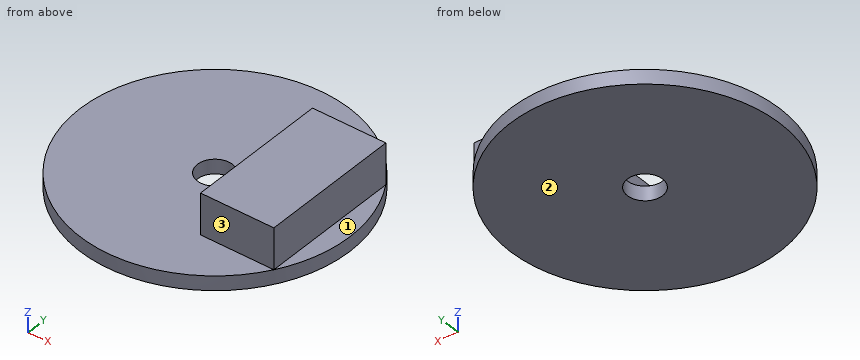
from build123d import *

# Parameters (mm, degrees)
SKETCH1_R           = 11.5
BOSS_EXTRUDE1_DEPTH = 1.23
SKETCH2_W           = 6.25
SKETCH2_H           = 12.059402844
BOSS_EXTRUDE2_DEPTH = 3.5
SKETCH3_R           = 1.5
CUT_EXTRUDE1_DEPTH  = 17.63580476


with BuildPart() as part:
    # Sketch1 → Boss-Extrude1 (new body)
    with BuildSketch(Plane.XY):
        Circle(SKETCH1_R)
    extrude(amount=BOSS_EXTRUDE1_DEPTH)

    # Sketch2 → Boss-Extrude2 (add)
    with BuildSketch(Plane.XY.offset(1.23)):
        with Locations((6.667481849, 0)):
            Rectangle(SKETCH2_W, SKETCH2_H)
    extrude(amount=BOSS_EXTRUDE2_DEPTH)

    # Sketch3 → Cut-Extrude1 (cut, through all)
    with BuildSketch(Plane.XY.offset(1.23)):
        Circle(SKETCH3_R)
    extrude(amount=-CUT_EXTRUDE1_DEPTH, mode=Mode.SUBTRACT)


solid = part.part
Here's how the part is built. I have some questions about the finished solid (model axes, mm). Face numbers are marked on the shaded views. A direction names the side the tool comes from. Coordinates: 2 decimals unless noted, no trailing zeros. Order: outer loops, then holes, each group sorted by start corner. A loop starts at its lowest first (then second) coordinate and runs counter-clockwise, first axis right, second up.
Item 1: If we section it at D-D on y = -3.75: List the corners of the cut face in (x, z) for me, plus the area to 3 significant figures.
Result sheet:
outline: (-10.87, 0) - (10.87, 0) - (10.87, 1.23) - (9.79, 1.23) - (9.79, 4.73) - (3.54, 4.73) - (3.54, 1.23) - (-10.87, 1.23) - close
area: 48.6 mm2
Item 2: If we section it at A-A on x = 0: List the corners of the cut face in (y, z) for me.
Result sheet:
outline: (-11.5, 0) - (-1.5, 0) - (-1.5, 1.23) - (-11.5, 1.23) - close; (1.5, 0) - (11.5, 0) - (11.5, 1.23) - (1.5, 1.23) - close
Item 3: If we section it at C-C on z = 0.55: List the corners of the cut face in (x, y) for me.
Result sheet:
outline: circle Ø23 at (0, 0); hole circle Ø3 at (0, 0)
Item 4: If we section it at B-B on y = 0: List the corners of the cut face in (x, z) for me.
Result sheet:
outline: (-11.5, 0) - (-1.5, 0) - (-1.5, 1.23) - (-11.5, 1.23) - close; (1.5, 0) - (11.5, 0) - (11.5, 1.23) - (9.79, 1.23) - (9.79, 4.73) - (3.54, 4.73) - (3.54, 1.23) - (1.5, 1.23) - close
Item 5: For P1, Ø1, axis at x = 7, z = 2.5, coming from the -Y side; P2, Ø12, axis at x = 8.5, y = -9, coming from the -Z side; P3, Ø0.9, axis at x = 11, y = 3, coming from the +Z side; P4, Ø2, axis at x = -4, z = 2, coming from the -Y side, each with a flat end and sliding along its axis, tell me the tip position at first contact or that it passes through.
Result sheet:
P1: stops at y = -6.03
P2: stops at z = 0
P3: stops at z = 1.23
P4: stops at y = -11
Item 6: For the marked faces 1, 2 and 3, which set-ups out of +Z, -Z, +X, -X, +Y, -Y let a thin tool reach every point of the face, with its end or its side?
Result sheet:
face 1: +Z, +X, +Y, -Y
face 2: -Z, +X, -X, +Y, -Y
face 3: +Z, +X, -X, -Y
Item 7: I need wall thicknesses on line 1 (Y direction, x = 0, z = 0.5); line 2 (Z direction, x = -5.75, y = -2.75); line 3 (Y direction, x = 7.25, z = 3.6). Which ranges of each line are inside material? Lowest first, please.
Result sheet:
line 1: y = -11.5 to -1.5, 1.5 to 11.5
line 2: z = 0 to 1.23
line 3: y = -6.03 to 6.03
